Input: part model. Units: mm. Frame: model coordinates. Coordinates: 2 decimals unless noted, no trailing zeros. Loops run counter-clockwise (first coordinate to the right, second up) from the corner with the lowest first, then second, coordinate; pieces in that order, holes last. Notation, with made-up numbers: (8.25, 39) -> (38.25, 39) arc R4 ccw to (38.25, 43) -> close; hole circle Ø6 at (-5, 31). An arc over 180 degrees is marked (long way). Put each result on its own line as item: value. Start each with the question number.
1) Material intervals for L1, parallel to X at y = -34.5, z = -6.5; L2, parallel to Z at x = -11.5, y = -54.5; L3, parallel to X at y = -52, z = -6, sorted ascending.
2) Contact query for flat-ended pins moving along their axis: P1, Ø12, axis at x = 23, y = -76.5, coming from the -Z side; P2, Ø6, axis at x = 7.5, y = -67.5, coming from the +Z side; P3, Ø6, axis at x = 19, y = -86.5, coming from the +Z side. Output: stop coordinate, or through.
3) Pull-direction query (X, two-part tool) for faces 1 (the cylindrical face through (-27.183, -51.511, -66.065)), 2 (the cylindrical face through (50.4, -51.51, 50.63)), 3 (the cylindrical face through (-50.4, -51.51, -50.63)); classes: pulls with the +X half, pulls with the -X half, needs draft (parallel to the pull), parting line crosses it, or undercut.
4) Cut plane A-A (z = 0). Return the cut outline in (x, y).
5) Cut plane C-C (x = -23.5). Return the cut outline in (y, z), plus the area to 3 significant figures.
from build123d import *

# Parameters (mm, degrees)
F0_R     = 76.2
F0_R_2   = 25.4
F1_DEPTH = 101.6
F3_DEPTH = 101.6


with BuildPart() as f1:
    # F0 (on Front) → F1 (new body)
    with BuildSketch(Plane.XZ):
        Circle(F0_R)
        Circle(F0_R_2, mode=Mode.SUBTRACT)
    extrude(amount=F1_DEPTH)

    # F2 (on face) → F3 (cut)
    with BuildSketch(Plane.XZ.offset(101.6)):
        with BuildLine():
            ThreePointArc((39.0757230448, 65.4181004656), (29.1604775462, 70.3996203774), (18.6268737068, 73.8882911963))
            ThreePointArc((18.6268737068, 73.8882911963), (27.3379476996, 65.9996441038), (39.0757230448, 65.4181004656))
        make_face()
        with BuildLine():
            ThreePointArc((61.1356839641, 45.484812259), (53.8815367264, 53.8815367264), (45.484812259, 61.1356839641))
            ThreePointArc((45.484812259, 61.1356839641), (50.513940681, 50.513940681), (61.1356839641, 45.484812259))
        make_face()
        with BuildLine():
            ThreePointArc((73.8882911963, 18.6268737068), (70.3996203774, 29.1604775462), (65.4181004656, 39.0757230448))
            ThreePointArc((65.4181004656, 39.0757230448), (65.9996441038, 27.3379476996), (73.8882911963, 18.6268737068))
        make_face()
        with BuildLine():
            ThreePointArc((76.2, 0), (75.9977505688, 5.5481445982), (75.3920758929, 11.0668375142))
            ThreePointArc((75.3920758929, 11.0668375142), (71.4375, 0), (75.3920758929, -11.0668375142))
            ThreePointArc((75.3920758929, -11.0668375142), (75.9977505688, -5.5481445982), (76.2, 0))
        make_face()
        with BuildLine():
            ThreePointArc((65.4181004656, -39.0757230448), (70.3996203774, -29.1604775462), (73.8882911963, -18.6268737068))
            ThreePointArc((73.8882911963, -18.6268737068), (65.9996441038, -27.3379476996), (65.4181004656, -39.0757230448))
        make_face()
        with BuildLine():
            ThreePointArc((45.484812259, -61.1356839641), (53.8815367264, -53.8815367264), (61.1356839641, -45.484812259))
            ThreePointArc((61.1356839641, -45.484812259), (50.513940681, -50.513940681), (45.484812259, -61.1356839641))
        make_face()
        with BuildLine():
            ThreePointArc((18.6268737068, -73.8882911963), (29.1604775462, -70.3996203774), (39.0757230448, -65.4181004656))
            ThreePointArc((39.0757230448, -65.4181004656), (27.3379476996, -65.9996441038), (18.6268737068, -73.8882911963))
        make_face()
        with BuildLine():
            ThreePointArc((11.0668375142, -75.3920758929), (0, -71.4375), (-11.0668375142, -75.3920758929))
            ThreePointArc((-11.0668375142, -75.3920758929), (0, -76.2), (11.0668375142, -75.3920758929))
        make_face()
        with BuildLine():
            ThreePointArc((-18.6268737068, -73.8882911963), (-27.3379476996, -65.9996441038), (-39.0757230448, -65.4181004656))
            ThreePointArc((-39.0757230448, -65.4181004656), (-29.1604775462, -70.3996203774), (-18.6268737068, -73.8882911963))
        make_face()
        with BuildLine():
            ThreePointArc((-45.484812259, -61.1356839641), (-50.513940681, -50.513940681), (-61.1356839641, -45.484812259))
            ThreePointArc((-61.1356839641, -45.484812259), (-53.8815367264, -53.8815367264), (-45.484812259, -61.1356839641))
        make_face()
        with BuildLine():
            ThreePointArc((-65.4181004656, -39.0757230448), (-65.9996441038, -27.3379476996), (-73.8882911963, -18.6268737068))
            ThreePointArc((-73.8882911963, -18.6268737068), (-70.3996203774, -29.1604775462), (-65.4181004656, -39.0757230448))
        make_face()
        with BuildLine():
            ThreePointArc((-75.3920758929, -11.0668375142), (-71.4375, 0), (-75.3920758929, 11.0668375142))
            ThreePointArc((-75.3920758929, 11.0668375142), (-76.2, 0), (-75.3920758929, -11.0668375142))
        make_face()
        with BuildLine():
            ThreePointArc((-73.8882911963, 18.6268737068), (-65.9996441038, 27.3379476996), (-65.4181004656, 39.0757230448))
            ThreePointArc((-65.4181004656, 39.0757230448), (-70.3996203774, 29.1604775462), (-73.8882911963, 18.6268737068))
        make_face()
        with BuildLine():
            ThreePointArc((-61.1356839641, 45.484812259), (-50.513940681, 50.513940681), (-45.484812259, 61.1356839641))
            ThreePointArc((-45.484812259, 61.1356839641), (-53.8815367264, 53.8815367264), (-61.1356839641, 45.484812259))
        make_face()
        with BuildLine():
            ThreePointArc((-39.0757230448, 65.4181004656), (-27.3379476996, 65.9996441038), (-18.6268737068, 73.8882911963))
            ThreePointArc((-18.6268737068, 73.8882911963), (-29.1604775462, 70.3996203774), (-39.0757230448, 65.4181004656))
        make_face()
        with BuildLine():
            Line((0, 76.2), (0, 71.4375))
            ThreePointArc((0, 71.4375), (5.8760863476, 72.455836431), (11.0668375142, 75.3920758929))
            ThreePointArc((11.0668375142, 75.3920758929), (5.5481445982, 75.9977505688), (0, 76.2))
        make_face()
        with BuildLine():
            ThreePointArc((-11.0668375142, 75.3920758929), (-5.8760863476, 72.455836431), (0, 71.4375))
            Line((0, 71.4375), (0, 76.2))
            ThreePointArc((0, 76.2), (-5.5481445982, 75.9977505688), (-11.0668375142, 75.3920758929))
        make_face()
    extrude(amount=-F3_DEPTH, mode=Mode.SUBTRACT)


solid = f1.part
Results found:
1. L1: x = -72.69 to -24.55, 24.55 to 72.69
1. L2: z = -75.33 to -22.65, 22.65 to 75.33
1. L3: x = -72.5 to -24.68, 24.68 to 72.5
2. P1: stops at z = -74.28
2. P2: stops at z = 74.95
2. P3: stops at z = 74.5
3. face 1: undercut
3. face 2: pulls with the +X half
3. face 3: pulls with the -X half
4. outline: (-71.44, -101.6) -> (-25.4, -101.6) -> (-25.4, 0) -> (-71.44, 0) -> close; (25.4, -101.6) -> (71.44, -101.6) -> (71.44, 0) -> (25.4, 0) -> close
5. outline: (-101.6, -68.2) -> (0, -68.2) -> (0, -9.64) -> (-101.6, -9.64) -> close; (-101.6, 9.64) -> (0, 9.64) -> (0, 68.2) -> (-101.6, 68.2) -> close
5. area: 11,900 mm2
